Could you check a few things on this model? Use its own coordinates, in mm. Face numbers are marked on the shaded views. Give positions to 0.01 mm unless a question says otherwise; leave off trailing zeros. Order: outer loops, then holes, each group sorted by start corner. A loop starts at its lowest first (then second) coordinate and runs counter-clockwise, first axis right, second up.
(1) Will these pins go through, and if not, where does the flat tip stop? pin 1 (5 mm diameter, centred on y = -4.5, z = -10.5, fed in from +X); pin 2 (4 mm diameter, centred on x = 10, y = -7.5, fed in from -Z); pin 3 (1.5 mm diameter, centred on x = 1.5, z = -2.5, fed in from +Y); pin 4 (2 mm diameter, centred on x = -6, z = -3, fed in from -Y).
(2) Imagine slicing it at D-D, the plane y = -8. Write out the boundary of the cut face in (x, z).
(3) Imagine slicing it at A-A, the plane x = 0. Write out the boundary of the cut face in (y, z).
(4) If we mould it in two halves opening along Z, with no side actions, what happens to the marked faces 1, 2, 3 and 4? For each: released by +Z, released by -Z, zero draft, split by the parting line, or undercut.
(5) Imagine slicing it at C-C, the plane y = -4.5. Write out the boundary of the cut face in (x, z), then the cut area to 3 significant figures.
(6) Imagine slicing it at B-B, the plane z = 0. Write out the boundary of the cut face in (x, y), then the cut area to 3 significant figures.
(7) If I drill on probe 1 along Z at (x, y) = (0, -0.85) (3 decimals); probe 2 along Y at (x, z) = (9, 2.25); probe 3 along Z at (x, y) = (0, -3.75) (3 decimals), over which ranges is the centre line in solid material (lowest first)?
from build123d import *

# Parameters (mm, degrees)
CROQUIS2_R            = 2.55
CORTAR_EXTRUIR1_DEPTH = 10
CROQUIS3_R            = 10
CORTAR_EXTRUIR2_DEPTH = 8


with BuildPart() as part:
    # Croquis1 → Revolución1 (revolve)
    with BuildSketch(Plane.XY):
        Polygon((-12.044691582, 0), (-15, 0), (-12, -10), (0, -10), (0, 0), align=None)
    revolve(axis=Axis((0, 0, 0), (0, -1, 0)))

    # Croquis2 → Cortar-Extruir1 (cut)
    with BuildSketch(Plane(origin=(0, 0, 0), x_dir=(1, 0, 0), z_dir=(0, 1, 0))):
        Circle(CROQUIS2_R)
    extrude(amount=-CORTAR_EXTRUIR1_DEPTH, mode=Mode.SUBTRACT)

    # Croquis3 → Cortar-Extruir2 (cut)
    with BuildSketch(Plane(origin=(0, -10, 0), x_dir=(-1, 0, 0), z_dir=(0, -1, 0))):
        Circle(CROQUIS3_R)
    extrude(amount=-CORTAR_EXTRUIR2_DEPTH, mode=Mode.SUBTRACT)


solid = part.part
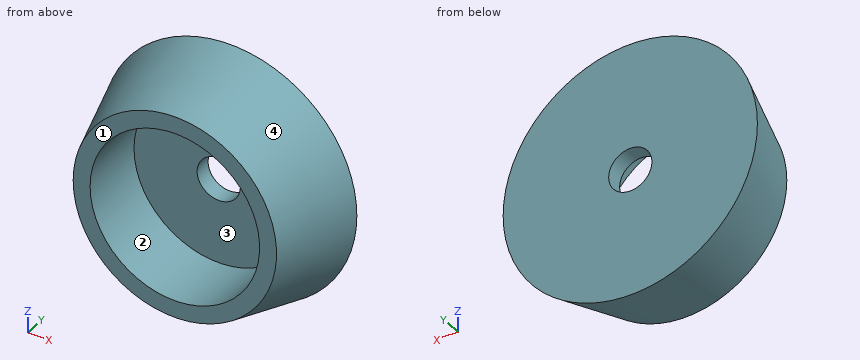
Answer block:
1. pin 1: stops at x = 11.28
1. pin 2: stops at z = -10.1
1. pin 3: stops at y = 0
1. pin 4: stops at y = -2
2. outline: circle Ø25.2 at (0, 0); hole circle Ø20 at (0, 0)
3. outline: (-10, -12) - (0, -15) - (0, -2.55) - (-2, -2.55) - (-2, -10) - (-10, -10) - close; (-10, 10) - (-2, 10) - (-2, 2.55) - (0, 2.55) - (0, 15) - (-10, 12) - close
4. face 1: zero draft
4. face 2: undercut
4. face 3: undercut
4. face 4: split by the parting line
5. outline: circle Ø27.3 at (0, 0); hole circle Ø20 at (0, 0)
5. area: 271 mm2
6. outline: (-15, 0) - (-12, -10) - (-10, -10) - (-10, -2) - (-2.55, -2) - (-2.55, 0) - close; (2.55, -2) - (10, -2) - (10, -10) - (12, -10) - (15, 0) - (2.55, 0) - close
6. area: 99.8 mm2
7. probe 1: z = -14.745 to -2.55, 2.55 to 14.745
7. probe 2: y = -2 to 0
7. probe 3: z = -13.875 to -10, 10 to 13.875
